```python
from build123d import *

# Parameters (mm, degrees)
SKETCH1_W           = 45
SKETCH1_H           = 20
BOSS_EXTRUDE1_DEPTH = 1
SKETCH2_R           = 8
SKETCH2_R_2         = 7
BOSS_EXTRUDE2_DEPTH = 12
BOSS_EXTRUDE3_DEPTH = 2
SKETCH5_R           = 1
SKETCH5_R_2         = 0.915040835
BOSS_EXTRUDE4_DEPTH = 1
SKETCH6_R           = 0.5
CUT_EXTRUDE1_DEPTH  = 1


with BuildPart() as part:
    # Sketch1 → Boss-Extrude1 (new body)
    with BuildSketch(Plane.XY):
        with Locations((0.550271739, 0.394021739)):
            Rectangle(SKETCH1_W, SKETCH1_H)
    extrude(amount=BOSS_EXTRUDE1_DEPTH)

    # Sketch2 → Boss-Extrude2 (add)
    # profile 1 of 2: a face of its own
    with BuildSketch(Plane.XY.offset(1)):
        with Locations((-12.452884101, 0.394021739)):
            Circle(SKETCH2_R)
        with Locations((-12.398133971, 0.339271609)):
            Circle(SKETCH2_R_2, mode=Mode.SUBTRACT)
    # profile 2 of 2: a face of its own
    with BuildSketch(Plane.XY.offset(1)):
        with Locations((13.547115899, 0.394021739)):
            Circle(SKETCH2_R)
        with Locations((13.55342758, 0.22977135)):
            Circle(SKETCH2_R_2, mode=Mode.SUBTRACT)
    extrude(amount=BOSS_EXTRUDE2_DEPTH)

    # Sketch4 → Boss-Extrude3 (add)
    with BuildSketch(Plane.XY.offset(1)):
        with BuildLine():
            Line((-2.6309647, 8.704551111), (5.3690353, 8.704551111))
            ThreePointArc((5.3690353, 8.704551111), (6.3690353, 7.704551111), (5.3690353, 6.704551111))
            Line((5.3690353, 6.704551111), (-2.6309647, 6.704551111))
            ThreePointArc((-2.6309647, 6.704551111), (-3.6309647, 7.704551111), (-2.6309647, 8.704551111))
        make_face()
    extrude(amount=BOSS_EXTRUDE3_DEPTH)

    # Sketch5 → Boss-Extrude4 (add)
    with BuildSketch(Plane.XY.offset(1)):
        with Locations((-3.619683348, -7.600525734)):
            Circle(SKETCH5_R)
        with Locations((-1.119683348, -7.600525734)):
            Circle(SKETCH5_R)
        with Locations((1.380316652, -7.600525734)):
            Circle(SKETCH5_R)
        with Locations((3.880316652, -7.600525734)):
            Circle(SKETCH5_R_2)
    extrude(amount=BOSS_EXTRUDE4_DEPTH)

    # Sketch6 → Cut-Extrude1 (cut)
    with BuildSketch(Plane.XY.offset(1)):
        with Locations((-20.209689263, 8.394021739)):
            Circle(SKETCH6_R)
        with Locations((21.050271739, -7.605978261)):
            Circle(SKETCH6_R)
    extrude(amount=-CUT_EXTRUDE1_DEPTH, mode=Mode.SUBTRACT)


solid = part.part
```
Verification items for the finished model (mm, model axes). A direction names the side the tool comes from. Coordinates: 2 decimals unless noted, no trailing zeros. Write each loop counter-clockwise with the first axis right and the second up, starting at its lowest first coordinate (ties: lowest second). Pieces come first, ordered by that corner, then holes. Notation, with made-up numbers: (38.5, 6.5) - (44.5, 6.5) arc R16 cw to (44.5, 16.5) - close; hole circle Ø9 at (-24.75, 88). An arc over 180 degrees is marked (long way). Write item = value, one per line.
Q1. Cross-section at A-A (z = 1.5). Give the number of separate pieces and of enclosed holes in the cut face, plus the area to 3 significant figures.
Answer:
separate_pieces = 7
enclosed_holes = 2
area = 125 mm²
Q2. Go/stop test with flat-tipped pins: pin 1 Ø3 at (x, z) = (-12, 4) entering from +Y; pin 2 Ø3 at (y, z) = (1, 9) entering from -X; pin 3 Ø2 at (x, y) = (1.5, -7.5) entering from +Z. Record where each tip stops, or that it passes through.
Answer:
pin_1 = 8.39
pin_2 = -20.45
pin_3 = 2
Q3. Mould release check, pull along X, two halves, no side actions. Record for faces 4 (the face through (1, 6.705, 2)), 5 (the face through (1, 8.705, 2)), 6 (the face through (-21.95, 0.3, 0.5)), 7 (the face through (-19.73, 8.54, 0.51)): released by +X, released by -X, zero draft, split by the parting line, or undercut.
Answer:
face_4 = undercut
face_5 = zero draft
face_6 = released by -X
face_7 = undercut
Q4. Material ranges on L1, parallel to X at y = 0, z = 8.5; L2, parallel to X at y = 2.5, z = 11; L3, parallel to Z at x = 10, y = 8.5, recorded low to high. Write a range as from..to.
Answer:
L1 = -20.44..-19.39, -5.41..-4.46, 5.56..6.56, 20.55..21.54
L2 = -20.17..-19.06, -5.74..-4.74, 5.83..6.93, 20.18..21.26
L3 = 0..1
Q5. Cross-section at D-D (z = 6.25). Enter the section's corners in (x, y).
Answer:
outline = circle Ø16 at (-12.45, 0.39); circle Ø16 at (13.55, 0.39); hole circle Ø14 at (-12.4, 0.34); hole circle Ø14 at (13.55, 0.23)
Q6. Cross-section at B-B (x = 7). Enter the section's corners in (y, z).
Answer:
outline = (-9.61, 0) - (10.39, 0) - (10.39, 1) - (4.99, 1) - (4.99, 13) - (2.69, 13) - (2.69, 1) - (-2.23, 1) - (-2.23, 13) - (-4.2, 13) - (-4.2, 1) - (-9.61, 1) - close
Q7. Access from +Z, -Z, +X, -X, +Y, -Y to the whole of each face (thin tool, end or side, straight path). Record for faces 1 (the face through (0.2, -9.606, 0.5)), 2 (the face through (-4, -8, 2)), 3 (the face through (-3.836, -8.577, 1.493)).
Answer:
face_1 = +Z, -Z, +X, -X, -Y
face_2 = +Z, -Y
face_3 = +Z
Q8. Cross-section at C-C (y = -4.25). Enter the section's corners in (x, z).
Answer:
outline = (-21.95, 0) - (23.05, 0) - (23.05, 1) - (20.06, 1) - (20.06, 13) - (18.93, 13) - (18.93, 1) - (8.17, 1) - (8.17, 13) - (7.03, 13) - (7.03, 1) - (-5.94, 1) - (-5.94, 13) - (-7.11, 13) - (-7.11, 1) - (-17.68, 1) - (-17.68, 13) - (-18.97, 13) - (-18.97, 1) - (-21.95, 1) - close
